from build123d import *

# Parameters (mm, degrees)
F1_DEPTH = 5


with BuildPart() as f1:
    # F0 (on Front) → F1 (new body)
    with BuildSketch(Plane.XZ):
        Polygon((952.385604, 1377.7951), (44.032343, 800.097644), (44.032343, 146.387324), (952.385604, 731.812539), align=None)
        Polygon((86.542191, 219.605512), (83.939075, 773.493111), (910.578549, 1311.283827), (910.578549, 750.689268), align=None, mode=Mode.SUBTRACT)
    extrude(amount=F1_DEPTH)


solid = f1.part
Geometry check sheet. Reference: the model listing, model coordinates, mm. A direction names the side the tool comes from. Round coordinates to 2 decimals unless told otherwise and drop trailing zeros. Loops run counter-clockwise (first coordinate to the right, second up) from the corner with the lowest first, then second, coordinate; pieces in that order, holes last. Notation, with made-up numbers: (-38.5, 52.5) -> (-3.5, 52.5) arc R33 ccw to (-3.5, 87.5) -> close; hole circle Ø7 at (12.5, 28). An arc over 180 degrees is marked (long way). Answer as a JSON object with one key per item and string values. Group by question number.
Item 1: Release check for a two-part mould opening along Y. For faces 1 (the face through (491.85, -2.46, 435)), 2 (the face through (664, 0, 583)), 3 (the face through (664, -5, 583)) record: pulls with the +Y half, pulls with the -Y half, needs draft (parallel to the pull), parting line crosses it, or undercut.
Item 2: Thickness scan on line 1 along Z through (x, y) = (377, -2.85); line 2 along Z through (x, y) = (714, -3.05); line 3 along X through (y, z) = (-0.5, 383). Record the ranges inside material, lowest first.
Item 3: Depth check by flat-ended pin: pin 1 Ø3 at (y, z) = (-2.5, 668.5) entering from +X; pin 2 Ø2 at (x, y) = (791, -0.5) entering from +Z; pin 3 Ø1.5 at (y, z) = (-1.5, 946.5) entering from -X. Enter the tip coordinate at first touch or a pass-through.
Item 4: Cross-section at B-B, the plane x = 205.5. Record the cut outline in (y, z), plus the area to 3 significant figures.
Item 5: Cross-section at A-A, the plane y = -3.5. Record the cut outline in (x, z), plus the area to 3 significant figures.
Item 6: Cross-section at C-C, the plane z = 714.5. Record the cut outline in (x, y).
Item 7: Set-up check for faces 4 (the face through (491.472, -2.465, 1038.624)), 5 (the face through (504.57, -2.46, 1092.99)): record each of +Z, -Z, +X, -X, +Y, -Y from which the full face is reachable in a straight line by a thin tool's end or side.
Determined:
{
 "1": {"face 1": "needs draft", "face 2": "pulls with the +Y half", "face 3": "pulls with the -Y half"},
 "2": {"line 1": "z = 360.98 to 406.8, 964.15 to 1011.86", "line 2": "z = 578.18 to 624, 1183.39 to 1226.19", "line 3": "x = 44.03 to 85.77, 340.07 to 411.16"},
 "3": {"pin 1": "stops at x = 856.48", "pin 2": "stops at z = 1275.79", "pin 3": "stops at x = 273.05"},
 "4": {"outline": "(-5, 250.45) -> (0, 250.45) -> (0, 296.27) -> (-5, 296.27) -> close; (-5, 852.58) -> (0, 852.58) -> (0, 902.79) -> (-5, 902.79) -> close", "area": "480 mm²"},
 "5": {"outline": "(44.03, 146.39) -> (952.39, 731.81) -> (952.39, 1377.8) -> (44.03, 800.1) -> close; hole (83.94, 773.49) -> (86.54, 219.61) -> (910.58, 750.69) -> (910.58, 1311.28) -> close", "area": "130,000 mm²"},
 "6": {"outline": "(44.03, -5) -> (84.22, -5) -> (84.22, 0) -> (44.03, 0) -> close; (854.43, -5) -> (925.52, -5) -> (925.52, 0) -> (854.43, 0) -> close"},
 "7": {"face 4": "+Y, -Y", "face 5": "+Z, -X, +Y, -Y"}
}
